For this review, use the dimensioned drawing (mm, ordinates from the lowest corner) and the shaded views. A direction names the side the tool comes from. Give positions to 0.01 mm unless a question says otherwise; leave off trailing zeros. Loops run counter-clockwise (first coordinate to the right, second up) from the corner with the lowest first, then second, coordinate; pieces in that order, holes last. Notation, with made-up numbers: M 24,48.5 L 33,48.5 A14 cw 33,59.5 Z; hole C -32.5,10.5 d9. An arc over 180 degrees is marked long. Use CSV: the item, a comma, the result in double quotes. Start each with the question number.
1. Take a section at A-A, the plane x = 31.2. Write out the cut boundary in (y, z) (3 decimals), and give its area (3 significant figures).
2. The part is to be moulded in two halves that separate along X. For the marked faces 1, 2 and 3, say which applies: pulls with the +X half, pulls with the -X half, needs draft (parallel to the pull), parting line crosses it, or undercut.
3. Take a section at B-B, the plane y = 30. Write out the cut boundary in (x, z) (3 decimals).
4. Insertion check: P1, Ø17, axis at x = 59, y = 18, coming from the -Z side (3 decimals); P2, Ø13, axis at y = 28.575, z = 45, coming from the +X side (3 decimals); P3, Ø6, axis at x = 61.2, y = 28.575, coming from the +Z side. Each pin has a flat end and moves straight along its axis. Give the tip position at first contact, or say it passes through.
5. To check wall thickness, follow line 1 (Y direction, x = 31.2, z = 74.25) (3 decimals); line 2 (X direction, y = 26.5, z = 62) (3 decimals); line 3 (Z direction, x = 21, y = 11) (3 decimals). State the ranges of each line that lie inside material, in increasing order. Write a range as [from, to].
6. Take a section at C-C, the plane z = 15. Write out the cut boundary in (x, y) (3 decimals), and give its area (3 significant figures).
7. Tool access review of the marked faces 4 and 5: name each direction out of +Z, -Z, +X, -X, +Y, -Y from which nothing blocks a thin tool from reaching the whole face with its end or side.
8. Take a section at D-D, the plane z = 68. Write out the cut boundary in (x, y) (3 decimals).
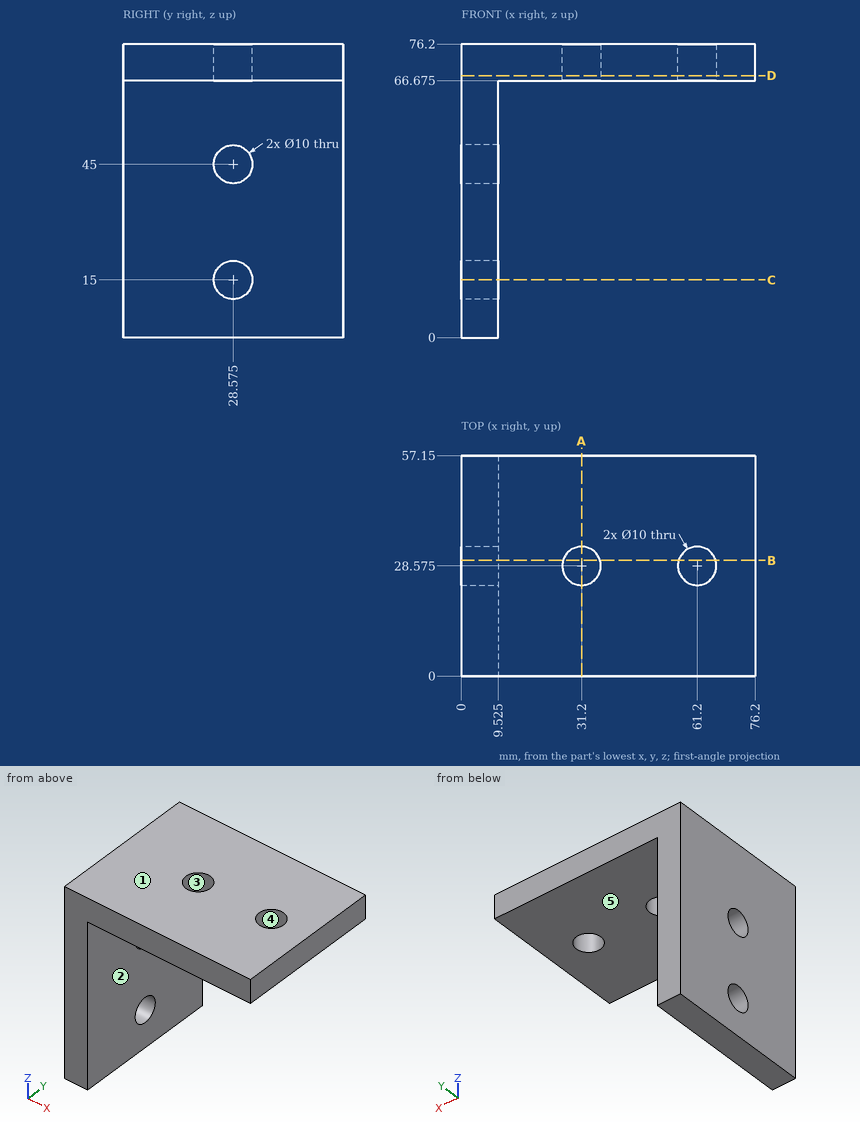
Result set:
1,outline,"M 0,66.675 L 23.575,66.675 L 23.575,76.2 L 0,76.2 Z; M 33.575,66.675 L 57.15,66.675 L 57.15,76.2 L 33.575,76.2 Z"
1,area,"449 mm2"
2,face 1,"needs draft"
2,face 2,"pulls with the +X half"
2,face 3,"undercut"
3,outline,"M 0,0 L 9.525,0 L 9.525,10.207 L 0,10.207 Z; M 0,19.793 L 9.525,19.793 L 9.525,40.207 L 0,40.207 Z; M 0,49.793 L 9.525,49.793 L 9.525,66.675 L 26.407,66.675 L 26.407,76.2 L 0,76.2 Z; M 35.993,66.675 L 56.407,66.675 L 56.407,76.2 L 35.993,76.2 Z; M 65.993,66.675 L 76.2,66.675 L 76.2,76.2 L 65.993,76.2 Z"
4,P1,"z = 66.675"
4,P2,"x = 9.525"
4,P3,"through"
5,line 1,"[0, 23.575], [33.575, 57.15]"
5,line 2,"[0, 9.525]"
5,line 3,"[66.675, 76.2]"
6,outline,"M 0,0 L 9.525,0 L 9.525,23.575 L 0,23.575 Z; M 0,33.575 L 9.525,33.575 L 9.525,57.15 L 0,57.15 Z"
6,area,"449 mm2"
7,face 4,"+Z, -Z"
7,face 5,"-Z, +X, +Y, -Y"
8,outline,"M 0,0 L 76.2,0 L 76.2,57.15 L 0,57.15 Z; hole C 31.2,28.575 d10; hole C 61.2,28.575 d10"
